Design review of the part shown in the three views and the two pictorial views. Dimensions are in mm from the part's minimum x, y and z. A direction names the side the tool comes from. Give positions to 0.01 mm unless a question says otherwise; leave off trailing zeros. Loops run counter-clockwise (first coordinate to the right, second up) from the corner with the lowest first, then second, coordinate; pieces in that order, holes last. Notation, with made-up numbers: (6.5, 39.5) -> (35.5, 39.5) arc R28 ccw to (35.5, 60.5) -> close; hole circle Ø11 at (-29, 67.25). An arc over 180 degrees is marked (long way). One line per question, with ' | ' between items. Start each with the question number.
(1) Consider section A-A (z = 150). Write out the cut boundary in (x, y).
(2) Wall thickness on probe 1 along Y at (x, z) = (322, 150); probe 2 along X at (y, z) = (350.5, 40.5); probe 3 along Y at (x, z) = (644, 239): over which ranges is each line inside the solid? List them lowest first.
(3) Consider section C-C (z = 56.5). Write out the cut boundary in (x, y).
(4) Tool access review of the marked faces 4, 5 and 6: name each direction out of +Z, -Z, +X, -X, +Y, -Y from which nothing blocks a thin tool from reaching the whole face with its end or side.
(5) Consider section B-B (y = 373). Write out the cut boundary in (x, z), and give its area (3 significant figures).
(6) Draft analysis for pull direction Z (two halves, no side actions). For the marked faces 1, 2 and 3, state which applies: +Z half, -Z half, draft (parallel to the pull), parting line (faces both ways), or undercut.
(7) Consider section D-D (x = 534). Write out the cut boundary in (y, z), and give its area (3 significant figures).
(8) Insertion check: P1, Ø6, axis at y = 45.5, z = 348.5, coming from the +X side; P2, Ø4, axis at x = 415.5, y = 163, coming from the -Z side; P3, Ø3, axis at x = 582, y = 86.5, coming from the +Z side; P4, Ø5, axis at x = 212.5, z = 318, coming from the +Y side. Each pin has a flat end and moves straight along its axis. Give the tip position at first contact, or say it passes through.
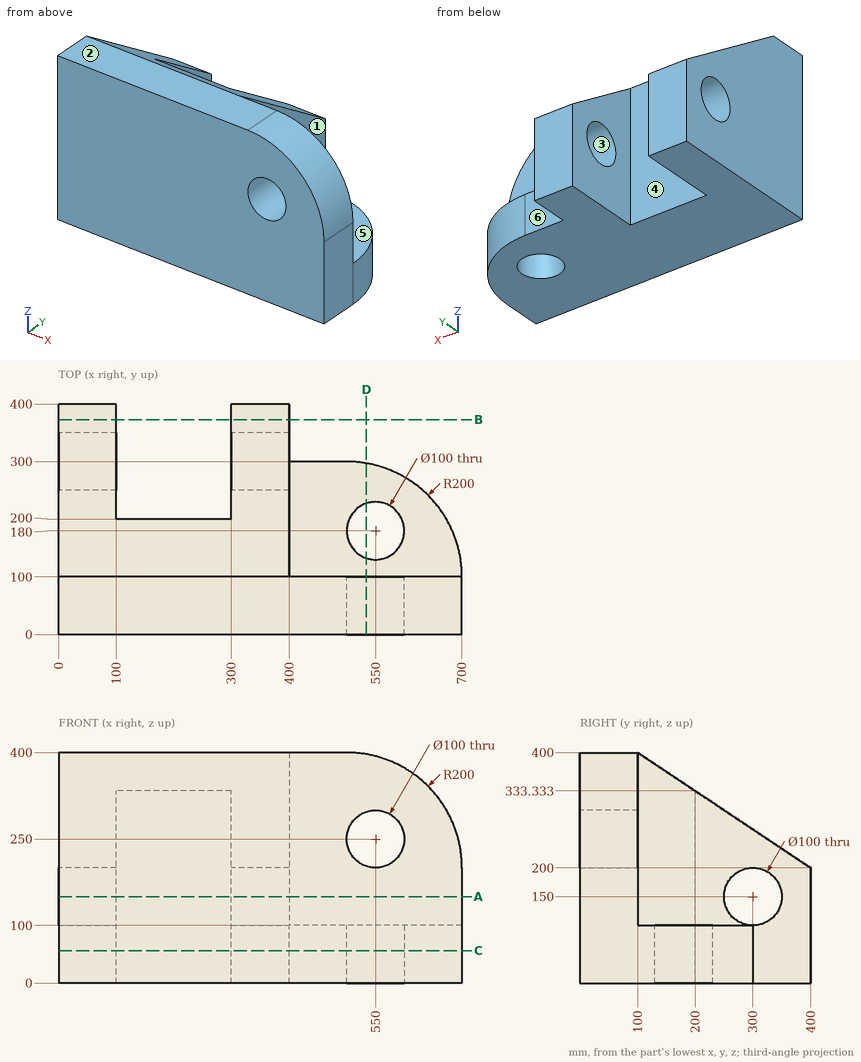
A:
1) outline: (0, 0) -> (700, 0) -> (700, 100) -> (400, 100) -> (400, 250) -> (300, 250) -> (300, 200) -> (100, 200) -> (100, 250) -> (0, 250) -> close; (0, 350) -> (100, 350) -> (100, 400) -> (0, 400) -> close; (300, 350) -> (400, 350) -> (400, 400) -> (300, 400) -> close
2) probe 1: y = 0 to 250, 350 to 400 | probe 2: x = 0 to 100, 300 to 400 | probe 3: y = 0 to 100
3) outline: (0, 0) -> (700, 0) -> (700, 100) arc R200 ccw to (500, 300) -> (400, 300) -> (400, 400) -> (300, 400) -> (300, 200) -> (100, 200) -> (100, 400) -> (0, 400) -> close; hole circle Ø100 at (550, 180)
4) face 4: +Z, -Z, +Y | face 5: +Z, +X, +Y | face 6: +Z, -Z, +X, +Y
5) outline: (0, 0) -> (100, 0) -> (100, 218) -> (0, 218) -> close; (300, 0) -> (400, 0) -> (400, 218) -> (300, 218) -> close | area: 43,600 mm^2
6) face 1: draft | face 2: +Z half | face 3: undercut
7) outline: (0, 0) -> (132.63, 0) -> (132.63, 100) -> (100, 100) -> (100, 202.63) -> (0, 202.63) -> close; (0, 297.37) -> (100, 297.37) -> (100, 397.09) -> (0, 397.09) -> close; (227.37, 0) -> (297.09, 0) -> (297.09, 100) -> (227.37, 100) -> close | area: 40,500 mm^2
8) P1: stops at x = 637.22 | P2: stops at z = 0 | P3: stops at z = 383.08 | P4: stops at y = 200
